from build123d import *

# Parameters (mm, degrees)
SKETCH1_R           = 24
SKETCH1_R_2         = 7.5
BOSS_EXTRUDE1_DEPTH = 70
BOSS_EXTRUDE3_DEPTH = 24
SKETCH3_R           = 7.5
CUT_EXTRUDE1_DEPTH  = 48
SKETCH4_R           = 15
CUT_EXTRUDE2_DEPTH  = 10
SKETCH5_R           = 15
CUT_EXTRUDE3_DEPTH  = 10
CUT_EXTRUDE4_DEPTH  = 20


with BuildPart() as part:
    # Sketch1 → Boss-Extrude1 (new body)
    with BuildSketch(Plane(origin=(0, 0, 0), x_dir=(1, 0, 0), z_dir=(0, 1, 0))):
        with Locations(Location((0, 0, 0), (0, 0, 270))):
            Circle(SKETCH1_R)
        with Locations(Location((0, 0, 0), (0, 0, 270))):
            Circle(SKETCH1_R_2, mode=Mode.SUBTRACT)
    extrude(amount=BOSS_EXTRUDE1_DEPTH)

    # Sketch2 → Boss-Extrude3 (add, symmetric)
    with BuildSketch(Plane(origin=(0, 0, 0), x_dir=(0, 0, -1), z_dir=(1, 0, 0))):
        Polygon((0, 55), (85, 55), (85, 115), (70, 115), (70, 70), (0, 70), align=None)
    extrude(amount=BOSS_EXTRUDE3_DEPTH, both=True)

    # Sketch3 → Cut-Extrude1 (cut)
    with BuildSketch(Plane(origin=(0, 55, 0), x_dir=(-1, 0, 0), z_dir=(0, -1, 0))):
        with Locations(Location((0, 0, 0), (0, 0, 270))):
            Circle(SKETCH3_R)
    extrude(amount=-CUT_EXTRUDE1_DEPTH, mode=Mode.SUBTRACT)

    # Sketch4 → Cut-Extrude2 (cut)
    with BuildSketch(Plane(origin=(0, 70, 0), x_dir=(1, 0, 0), z_dir=(0, 1, 0))):
        with Locations(Location((0, 0, 0), (0, 0, 270))):
            Circle(SKETCH4_R)
    extrude(amount=-CUT_EXTRUDE2_DEPTH, mode=Mode.SUBTRACT)

    # Sketch5 → Cut-Extrude3 (cut)
    with BuildSketch(Plane.XZ):
        with Locations(Location((0, 0, 0), (0, 0, 90))):
            Circle(SKETCH5_R)
    extrude(amount=-CUT_EXTRUDE3_DEPTH, mode=Mode.SUBTRACT)

    # Sketch6 → Cut-Extrude4 (cut)
    with BuildSketch(Plane(origin=(0, 0, -85), x_dir=(-1, 0, 0), z_dir=(0, 0, -1))):
        with BuildLine():
            Line((-8, 95), (-8, 115))
            Line((-8, 115), (8, 115))
            Line((8, 115), (8, 95))
            ThreePointArc((8, 95), (0, 87), (-8, 95))
        make_face()
    extrude(amount=-CUT_EXTRUDE4_DEPTH, mode=Mode.SUBTRACT)


solid = part.part
Work out the finished part from the listing and answer in its coordinate system (mm). A direction names the side the tool comes from. Round coordinates to 2 decimals unless told otherwise and drop trailing zeros. Write each loop counter-clockwise with the first axis right and the second up, starting at its lowest first coordinate (ties: lowest second). Pieces come first, ordered by that corner, then holes. Notation, with made-up numbers: (89, 33.5) -> (118, 33.5) arc R33 ccw to (118, 67.5) -> close; hole circle Ø2 at (-7.5, 65). An arc over 180 degrees is marked (long way). Answer as CSV lines item,"result". Start each with the question number.
(1) The part is cut by section C-C, the plane y = 106.5. Give the vertices of the cut face in (x, z), then the cut area to 3 significant figures.
(2) Find the intervals of material crossed by probe 1 along Z at (x, y) = (0, 32); probe 2 along X at (y, z) = (2, 0), in increasing order.
(3) The part is cut by section A-A, the plane x = 0. Give the vertices of the cut face in (y, z).
(4) Each of these flat-tipped pins is pushed along its axis until it touches: pin 1 (1.5 mm diameter, centred on x = -8, z = -18, fed in from -Y); pin 2 (3 mm diameter, centred on x = -18, z = -9.5, fed in from +Y); pin 3 (9 mm diameter, centred on x = 6, z = 3.5, fed in from -Y); pin 4 (2 mm diameter, centred on x = 15, y = 61.5, fed in from +Z). Where does it stop, or does it pass through?
(5) The part is cut by section D-D, the plane y = 83.5. Give the vertices of the cut face in (x, z).
(6) The part is cut by section B-B, the plane z = -4. Give the vertices of the cut face in (x, y).
(7) A tool of negligible diameter and unlimited length cuts with its end or side. For faces 5 (the flat face through (0, 70, -34)), 6 (the flat face through (7, 60, -4)), 7 (the flat face through (-8, 105, -78)), from which of +Z, -Z, +X, -X, +Y, -Y can it reach the whole face along a straight path? Write none if from no direction.
(8) The mould has two halves that part along Z. Classify faces 1 (the flat face through (-24, 65, -61)), 2 (the cylindrical face through (-0.66, 4.93, -14.985)), 3 (the flat face through (6, 88, -70)), 4 (the flat face through (0, 85, -85)): +Z half, -Z half, draft (parallel to the pull), parting line (faces both ways), or undercut.
Output values:
1,outline,"(-24, -85) -> (-8, -85) -> (-8, -70) -> (-24, -70) -> close; (8, -85) -> (24, -85) -> (24, -70) -> (8, -70) -> close"
1,area,"480 mm²"
2,probe 1,"z = -24 to -7.5, 7.5 to 24"
2,probe 2,"x = -24 to -15, 15 to 24"
3,outline,"(0, -24) -> (55, -24) -> (55, -85) -> (87, -85) -> (87, -70) -> (70, -70) -> (70, -15) -> (60, -15) -> (60, -7.5) -> (10, -7.5) -> (10, -15) -> (0, -15) -> close; (0, 15) -> (10, 15) -> (10, 7.5) -> (60, 7.5) -> (60, 15) -> (70, 15) -> (70, 24) -> (0, 24) -> close"
4,pin 1,"stops at y = 0"
4,pin 2,"stops at y = 70"
4,pin 3,"stops at y = 10"
4,pin 4,"stops at z = 19.49"
5,outline,"(-24, -85) -> (24, -85) -> (24, -70) -> (-24, -70) -> close"
6,outline,"(-24, 55) -> (-23.66, 55) -> (-23.66, 0) -> (-14.46, 0) -> (-14.46, 10) -> (-6.34, 10) -> (-6.34, 60) -> (-14.46, 60) -> (-14.46, 70) -> (-24, 70) -> close; (6.34, 10) -> (14.46, 10) -> (14.46, 0) -> (23.66, 0) -> (23.66, 55) -> (24, 55) -> (24, 70) -> (14.46, 70) -> (14.46, 60) -> (6.34, 60) -> close"
7,face 5,"+Z, +X, -X, +Y"
7,face 6,"+Y"
7,face 7,"+Z, -Z, +Y"
8,face 1,"draft"
8,face 2,"undercut"
8,face 3,"+Z half"
8,face 4,"-Z half"
